The listing builds one solid part. Answer for the finished solid, in the listing's coordinates (mm). Give positions to 0.01 mm unless a question says otherwise; leave off trailing zeros. Loops run counter-clockwise (first coordinate to the right, second up) from the corner with the lowest first, then second, coordinate; pieces in that order, holes last. Notation, with made-up numbers: M -31.5,64 L 6.5,64 A31 cw 6.5,103 Z; hole C 6,76 d2. An arc over 180 degrees is marked long. Use one line per item in the form item = value. Start each with the question number.
1. The part is cut by section A-A (x = 0). Write down the section's boundary in (y, z), and give its area (3 significant figures).
2. The part is cut by section D-D (x = 40.5). Write down the section's boundary in (y, z), and give its area (3 significant figures).
3. The part is cut by section B-B (z = 2.35). Write down the section's boundary in (x, y).
4. Straight lines are drawn through the part: line 1 (Y direction, x = 0, z = 2.4); line 2 (X direction, y = 23, z = 2.7); line 3 (X direction, y = 10, z = 2). For each, find the intervals that lie inside material, in ascending order. Write a range as from..to.
5. Each of these flat-tipped pins is pushed along its axis until it touches: pin 1 Ø1 at (x, z) = (41.5, 2) entering from +Y; pin 2 Ø1.5 at (y, z) = (-26.5, 1.5) entering from +X; pin 3 Ø5 at (x, y) = (53.26, -30.75) entering from +Z. Where does it stop, or does it pass through?
6. The part is cut by section C-C (y = 8.5). Write down the section's boundary in (x, z).
from build123d import *

# Parameters (mm, degrees)
F0_R     = 72
F1_DEPTH = 3
F2_R     = 25.5
F3_DEPTH = 3
F4_R     = 3
F4_R_2   = 4.5
F5_DEPTH = 25.4
F6_R     = 3
F7_DEPTH = 25.4


with BuildPart() as f1:
    # F0 (on Top) → F1 (new body)
    with BuildSketch(Plane.XY):
        Circle(F0_R)
    extrude(amount=F1_DEPTH)

    # F2 (on face) → F3 (cut)
    with BuildSketch(Plane.XY.offset(3)):
        with Locations((-40.5, 0)):
            Circle(F2_R)
        with Locations((40.5, 0)):
            Circle(F2_R)
    extrude(amount=-F3_DEPTH, mode=Mode.SUBTRACT)

    # F4 (on face) → F5 (cut)
    with BuildSketch(Plane.XY.offset(3)):
        with Locations((0, 61.5)):
            Circle(F4_R)
        Circle(F4_R_2)
        with Locations((0, -61.5)):
            Circle(F4_R)
    extrude(amount=-F5_DEPTH, mode=Mode.SUBTRACT)

    # F6 (on face) → F7 (cut)
    with BuildSketch(Plane.XY.offset(3)):
        with Locations((-53.260562, -30.75)):
            Circle(F6_R)
        with Locations((53.260562, -30.75)):
            Circle(F6_R)
    extrude(amount=-F7_DEPTH, mode=Mode.SUBTRACT)


solid = f1.part
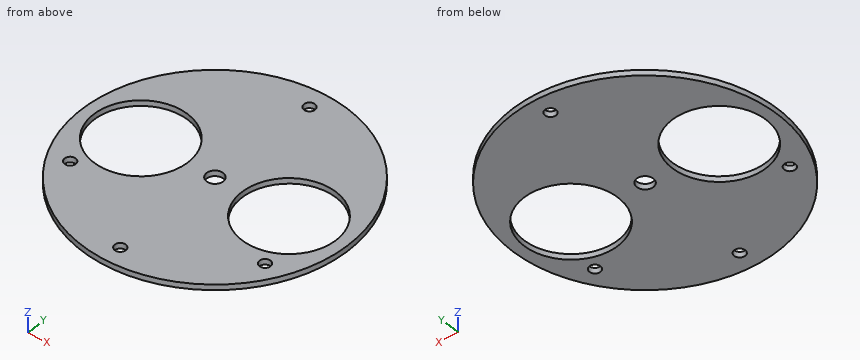
Derived:
q1.outline = M -72,0 L -64.5,0 L -64.5,3 L -72,3 Z; M -58.5,0 L -4.5,0 L -4.5,3 L -58.5,3 Z; M 4.5,0 L 58.5,0 L 58.5,3 L 4.5,3 Z; M 64.5,0 L 72,0 L 72,3 L 64.5,3 Z
q1.area = 369 mm2
q2.outline = M -59.53,0 L -25.5,0 L -25.5,3 L -59.53,3 Z; M 25.5,0 L 59.53,0 L 59.53,3 L 25.5,3 Z
q2.area = 204 mm2
q3.outline = C 0,0 d144; hole C -40.5,0 d51; hole C -53.26,-30.75 d6; hole C 0,0 d9; hole C 0,-61.5 d6; hole C 0,61.5 d6; hole C 40.5,0 d51; hole C 53.26,-30.75 d6
q4.line_1 = -72..-64.5, -58.5..-4.5, 4.5..58.5, 64.5..72
q4.line_2 = -68.23..-51.51, -29.49..29.49, 51.51..68.23
q4.line_3 = -71.3..-63.96, -17.04..17.04, 63.96..71.3
q5.pin_1 = 59.19
q5.pin_2 = 67.24
q5.pin_3 = through
q6.outline = M -71.5,0 L -64.54,0 L -64.54,3 L -71.5,3 Z; M -16.46,0 L 16.46,0 L 16.46,3 L -16.46,3 Z; M 64.54,0 L 71.5,0 L 71.5,3 L 64.54,3 Z
